Design review of the part built by this model. Coordinates are the model's own, in mm. A direction names the side the tool comes from. Coordinates: 2 decimals unless noted, no trailing zeros. Loops run counter-clockwise (first coordinate to the right, second up) from the corner with the lowest first, then second, coordinate; pieces in that order, holes last. Notation, with made-up numbers: (67.25, 70) - (93.25, 70) arc R15 ccw to (93.25, 98) - close; hole circle Ø6 at (-6, 0). An arc over 180 degrees is marked (long way). Answer in a Markdown table with one row per item. Add a question column.
(1) We need section A-A, the plane x = 3.25. Write out the cut boundary in (y, z).
(2) We need section D-D, the plane z = 2.4. Write out the cut boundary in (x, y), plus the area to 3 significant figures.
(3) The part is to be moulded in two halves that separate along X. For faces 1 (the face through (14, -16, 3)), 2 (the face through (12, -8, 3)), 3 (the face through (4.093, 1.521, 3.271)), 4 (the face through (16, -6, 3)), say which applies: released by +X, released by -X, zero draft, split by the parting line, or undercut.
(4) Clearance check with flat-ended pins moving along their axes: pin 1 (0.8 mm diameter, centred on y = 3.5, z = 2, fed in from -X); pin 2 (1.8 mm diameter, centred on x = 9, z = 3, fed in from -Y); pin 3 (3 mm diameter, centred on x = 4.5, z = 3, fed in from +Y). State where each tip first meets the part, or that it passes through.
(5) We need section C-C, the plane y = 1. Write out the cut boundary in (x, z), plus the area to 3 significant figures.
(6) To check wall thickness, follow L1, parallel to X at y = -4.75, z = 1.6; L2, parallel to Y at x = 3, z = 0.95; L3, parallel to X at y = 0.25, z = 3.05. State the ranges of each line that lie inside material, in increasing order. Write a range as [from, to].
(7) For faces 5 (the face through (6, 0, 3)), 6 (the face through (4, 3, 4)), 7 (the face through (13, -2, 6)), list the 3-axis set-ups (+Z, -Z, +X, -X, +Y, -Y) from which the entire face can be reached by the end or side of a thin tool; tool diameter is ignored.
(8) We need section B-B, the plane z = 1.45. Write out the cut boundary in (x, y), plus the area to 3 significant figures.
from build123d import *

# Parameters (mm, degrees)
SKETCH1_W           = 15
SKETCH1_H           = 6
BOSS_EXTRUDE1_DEPTH = 3
CUT_EXTRUDE1_REACH  = 18.432
SKETCH2_R           = 1
SKETCH3_W           = 3
SKETCH3_H           = 6
BOSS_EXTRUDE2_DEPTH = 16
SKETCH4_W           = 6
SKETCH4_H           = 19
BOSS_EXTRUDE3_DEPTH = 1
SKETCH5_W           = 8
SKETCH5_H           = 6
BOSS_EXTRUDE4_DEPTH = 1


with BuildPart() as part:
    # Sketch1 → Boss-Extrude1 (new body)
    with BuildSketch(Plane(origin=(0, 0, 0), x_dir=(1, 0, 0), z_dir=(0, 1, 0))):
        with Locations((7.5, -3)):
            Rectangle(SKETCH1_W, SKETCH1_H)
    extrude(amount=BOSS_EXTRUDE1_DEPTH)

    # Sketch2 → Cut-Extrude1 (cut, up to next)
    with BuildSketch(Plane(origin=(0, 3, 0), x_dir=(1, 0, 0), z_dir=(0, 1, 0)), mode=Mode.PRIVATE) as cut_extrude1_sk1:
        with Locations(Location((3.25, -2.733160164, 0), (0, 0, 270))):
            Circle(SKETCH2_R)
    cut_extrude1_tool1 = extrude(cut_extrude1_sk1.sketch, amount=-CUT_EXTRUDE1_REACH, mode=Mode.PRIVATE) & part.part
    add(cut_extrude1_tool1.solids().sort_by_distance((3.25, 3, 2.73316))[0], mode=Mode.SUBTRACT)

    # Sketch3 → Boss-Extrude2 (add)
    with BuildSketch(Plane.XZ):
        with Locations((13.5, 3)):
            Rectangle(SKETCH3_W, SKETCH3_H)
    extrude(amount=BOSS_EXTRUDE2_DEPTH)

    # Sketch4 → Boss-Extrude3 (add)
    with BuildSketch(Plane(origin=(15, 0, 0), x_dir=(0, 0, -1), z_dir=(1, 0, 0))):
        with Locations((-3, -6.5)):
            Rectangle(SKETCH4_W, SKETCH4_H)
    extrude(amount=BOSS_EXTRUDE3_DEPTH)

    # Sketch5 → Boss-Extrude4 (add)
    with BuildSketch(Plane(origin=(0, 3, 0), x_dir=(1, 0, 0), z_dir=(0, 1, 0))):
        with Locations((12, -3)):
            Rectangle(SKETCH5_W, SKETCH5_H)
    extrude(amount=BOSS_EXTRUDE4_DEPTH)


solid = part.part
Responses:
| question | item | result |
|---|---|---|
| 1 | outline | (0, 0) - (3, 0) - (3, 1.73) - (0, 1.73) - close; (0, 3.73) - (3, 3.73) - (3, 6) - (0, 6) - close |
| 2 | outline | (0, 0) - (2.31, 0) - (2.31, 3) - (0, 3) - close; (4.19, 0) - (12, 0) - (12, -16) - (16, -16) - (16, 4) - (8, 4) - (8, 3) - (4.19, 3) - close |
| 2 | area | 114 mm2 |
| 3 | face 1 | zero draft |
| 3 | face 2 | released by -X |
| 3 | face 3 | undercut |
| 3 | face 4 | released by +X |
| 4 | pin 1 | stops at x = 8 |
| 4 | pin 2 | stops at y = 0 |
| 4 | pin 3 | stops at y = 3 |
| 5 | outline | (0, 0) - (16, 0) - (16, 6) - (0, 6) - close; hole circle Ø2 at (3.25, 2.73) |
| 5 | area | 92.9 mm2 |
| 6 | L1 | x = [12, 16] |
| 6 | L2 | y = [0, 3] |
| 6 | L3 | x = [0, 2.3], [4.2, 16] |
| 7 | face 5 | +Z, -Z, -X, -Y |
| 7 | face 6 | +Z, -Z, -X, +Y |
| 7 | face 7 | +Z, +X, -X, +Y, -Y |
| 8 | outline | (0, 0) - (12, 0) - (12, -16) - (16, -16) - (16, 4) - (8, 4) - (8, 3) - (0, 3) - close |
| 8 | area | 120 mm2 |
